Work out the finished part from the listing and answer in its coordinate system (mm). A direction names the side the tool comes from. Coordinates: 2 decimals unless noted, no trailing zeros. Write each loop counter-clockwise with the first axis right and the second up, starting at its lowest first coordinate (ties: lowest second). Pieces come first, ordered by that corner, then holes. Notation, with made-up numbers: (-18, -9.75) - (-8, -9.75) arc R20 ccw to (-8, 9.25) - close; hole circle Ø5 at (77.5, -2.5). An arc over 180 degrees is marked (long way). Use CSV: the item, a comma, the result in double quotes. Start each with the question number.
from build123d import *

# Parameters (mm, degrees)
SKETCH2_W               = 60
SKETCH2_H               = 82
BOSS_EXTRUDE2_DEPTH     = 10
SKETCH4_R               = 20
BOSS_EXTRUDE3_DEPTH     = 60
SKETCH8_W               = 50
SKETCH8_H               = 50
CUT_EXTRUDE1_DEPTH      = 50
CUT_EXTRUDE2_DEPTH      = 50
SKETCH14_W              = 40
SKETCH14_H              = 23.219607056
CUT_EXTRUDE3_DEPTH      = 3
CUT_EXTRUDE4_REACH      = 114.236
CUT_EXTRUDE4_END_RADIUS = 20
SKETCH15_R              = 5


with BuildPart() as part:
    # Sketch2 → Boss-Extrude2 (new body)
    with BuildSketch(Plane(origin=(0, 0, 0), x_dir=(1, 0, 0), z_dir=(0, 1, 0))):
        Rectangle(SKETCH2_W, SKETCH2_H)
    extrude(amount=BOSS_EXTRUDE2_DEPTH)

    # Sketch4 → Boss-Extrude3 (add, through all)
    with BuildSketch(Plane(origin=(30, 0, 0), x_dir=(0, 0, -1), z_dir=(1, 0, 0))):
        with BuildLine():
            Line((41, 10), (-41, 10))
            Line((-41, 10), (20.123633203, 67.417511832))
            ThreePointArc((20.123633203, 67.417511832), (71.995026669, 62.794453129), (61.436533479, 11.799038106))
            Line((61.436533479, 11.799038106), (41, 0))
            Line((41, 0), (41, 10))
        make_face()
        with Locations((44, 42)):
            Circle(SKETCH4_R, mode=Mode.SUBTRACT)
    extrude(amount=-BOSS_EXTRUDE3_DEPTH)

    # Sketch8 → Cut-Extrude1 (cut)
    with BuildSketch(Plane(origin=(0, 60, 0), x_dir=(1, 0, 0), z_dir=(0, 1, 0))):
        with Locations((0, -16)):
            Rectangle(SKETCH8_W, SKETCH8_H)
    extrude(amount=-CUT_EXTRUDE1_DEPTH, mode=Mode.SUBTRACT)

    # Sketch9 → Cut-Extrude2 (cut)
    with BuildSketch(Plane(origin=(0, 10, 0), x_dir=(1, 0, 0), z_dir=(0, 1, 0))):
        with BuildLine():
            Line((-15, -21), (15, -21))
            ThreePointArc((15, -21), (20, -26), (15, -31))
            Line((15, -31), (-15, -31))
            ThreePointArc((-15, -31), (-20, -26), (-15, -21))
        make_face()
    extrude(amount=-CUT_EXTRUDE2_DEPTH, mode=Mode.SUBTRACT)

    # Sketch14 → Cut-Extrude3 (cut)
    with BuildSketch(Plane(origin=(0, 77, 0), x_dir=(1, 0, 0), z_dir=(0, 1, 0))):
        with Locations((0, 49.498350081)):
            Rectangle(SKETCH14_W, SKETCH14_H)
    extrude(amount=-CUT_EXTRUDE3_DEPTH, mode=Mode.SUBTRACT)

    # Cut-Extrude4: up to this cylinder (the profile starts outside it)
    cut_extrude4_end = Plane(origin=(0, 42, -44), z_dir=(1, 0, 0)) * Cylinder(CUT_EXTRUDE4_END_RADIUS, 269.472, mode=Mode.PRIVATE)
    # Sketch15 → Cut-Extrude4 (cut, up to the surface)
    with BuildSketch(Plane(origin=(0, 74, 0), x_dir=(1, 0, 0), z_dir=(0, 1, 0)), mode=Mode.PRIVATE) as cut_extrude4_sk1:
        with Locations(Location((0, 47.874836009, 0), (0, 0, 270))):
            Circle(SKETCH15_R)
    cut_extrude4_tool1 = extrude(cut_extrude4_sk1.sketch, amount=-CUT_EXTRUDE4_REACH, mode=Mode.PRIVATE) - cut_extrude4_end
    add(cut_extrude4_tool1.solids().sort_by_distance((0, 74, -47.874836))[0], mode=Mode.SUBTRACT)


solid = part.part
Item 1: A cutting plane is placed at B-B (z = 26). Determine the outline of the cut face in (x, y), then the cut area to 3 significant figures.
Item 2: Each of these flat-tipped pins is pushed along its axis until it touches: pin 1 (3 mm diameter, centred on x = -6, y = 30.5, fed in from -Z); pin 2 (11.5 mm diameter, centred on x = 0, z = -47.87, fed in from +Y); pin 3 (11 mm diameter, centred on x = -6, y = 6.5, fed in from -Z). Where does it stop, or does it pass through?
Item 3: A cutting plane is placed at A-A (x = -10). Determine the outline of the cut face in (y, z), then the cut area to 3 significant figures.
Item 4: A cutting plane is placed at C-C (y = 42). Determine the outline of the cut face in (x, z), then the cut area to 3 significant figures.
Item 5: Determine the mould class of faces 5 (the face through (0, 5, 21)), 6 (the face through (-30, 30, -20)), 7 (the face through (30, 30, -20)), 8 (the face through (20, 75, -46)) for opening direction X: +X half, -X half, draft (parallel to the pull), parting line (faces both ways), or undercut.
Item 6: Which of the six approach directions +Z, -Z, +X, -X, +Y, -Y give full straight-line access (tool end or side, diameter ignored) to faces 1 (the face through (0.22, 67.06, -52.87)), 2 (the face through (25, 23, 5)), 3 (the face through (0, 5, 31)), 4 (the face through (0, 75, -37.889))?
Item 7: Straight lines are drawn through the part: probe 1 along Y at (x, z) = (14, -51.5); probe 2 along X at (y, z) = (19.5, 15); probe 3 along Z at (x, y) = (8.5, 38.5). For each, find the intervals that lie inside material, in ascending order. Write a range as [from, to].
Item 8: A cutting plane is placed at D-D (x = 0). Determine the outline of the cut face in (y, z), then the cut area to 3 significant figures.
Calculated:
1,outline,"(-30, 0) - (-20, 0) - (-20, 10) - (-25, 10) - (-25, 24.09) - (-30, 24.09) - close; (20, 0) - (30, 0) - (30, 24.09) - (25, 24.09) - (25, 10) - (20, 10) - close"
1,area,"341 mm²"
2,pin 1,"stops at z = -77.41"
2,pin 2,"stops at y = 74"
2,pin 3,"stops at z = -61.78"
3,outline,"(0, -41) - (11.8, -61.44) arc R34.87 ccw to (74, -57.86) - (74, -37.89) - (76.33, -37.89) arc R34.87 ccw to (67.42, -20.12) - (56.97, -9) - (10, -9) - (10, 21) - (0, 21) - close; (0, 31) - (10, 31) - (10, 41) - (0, 41) - close; hole circle Ø40 at (42, -44)"
3,area,"3,500 mm²"
4,outline,"(-30, -78.87) - (30, -78.87) - (30, -64) - (-30, -64) - close; (-30, -24) - (30, -24) - (30, 6.93) - (25, 6.93) - (25, -9) - (-25, -9) - (-25, 6.93) - (-30, 6.93) - close"
4,area,"1,950 mm²"
5,face 5,"undercut"
5,face 6,"-X half"
5,face 7,"+X half"
5,face 8,"undercut"
6,face 1,"+Y"
6,face 2,"+Z, +Y"
6,face 3,"+Y, -Y"
6,face 4,"-Z, +Y"
7,probe 1,"y = [6.06, 23.46], [60.54, 74]"
7,probe 2,"x = [-30, -25], [25, 30]"
7,probe 3,"z = [-78.7, -63.69], [-24.31, -9]"
8,outline,"(0, -41) - (11.8, -61.44) arc R34.87 ccw to (74, -57.86) - (74, -52.87) - (59.92, -52.87) arc R20 cw (long way) to (61.97, -42.87) - (74, -42.87) - (74, -37.89) - (76.33, -37.89) arc R34.87 ccw to (67.42, -20.12) - (56.97, -9) - (10, -9) - (10, 21) - (0, 21) - close; (0, 31) - (10, 31) - (10, 41) - (0, 41) - close"
8,area,"3,370 mm²"
